Design review of the part built by this model. Coordinates are the model's own, in mm. Face numbers are marked on the shaded views. A direction names the side the tool comes from. Coordinates: 2 decimals unless noted, no trailing zeros. Write each loop counter-clockwise with the first axis right and the second up, starting at its lowest first coordinate (ties: lowest second). Pieces come first, ordered by that corner, then holes. Notation, with made-up numbers: M 12,62 L 17,62 A28 ccw 17,91 Z; hole C 82,-37.5 d6. An arc over 180 degrees is marked long. Return JSON: item names as keys, results as strings. Group by question number.
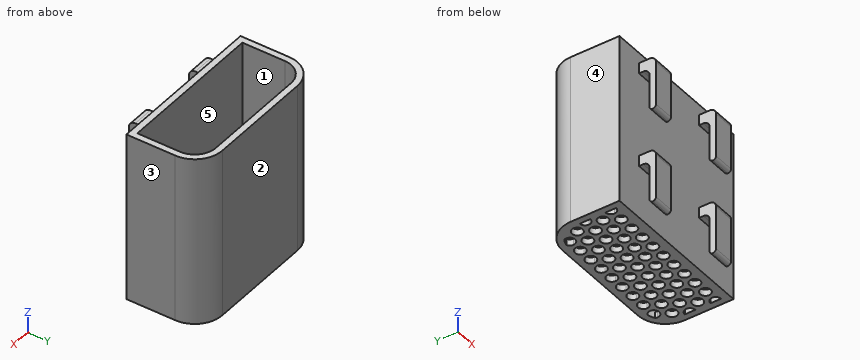
```python
from build123d import *

# Parameters (mm, degrees)
F1_DEPTH = 80
F2_DEPTH = 3
F3_R     = 2.5
F4_DEPTH = 3
F5_W     = 10
F5_H     = 5
F6_DEPTH = 5
F7_W     = 10
F7_H     = 25
F8_DEPTH = 3
F9_R     = 3
F10_R    = 1.49999


# Not quite as in the source:
# - a fillet or chamfer is up to 0.001 mm smaller than in the source, because OpenCascade refuses the exact size


with BuildPart() as f1:
    # F0 (on Top) → F1 (new body)
    with BuildSketch(Plane.XY):
        with BuildLine():
            Line((-38, 5), (-38, -18))
            Line((-38, -18), (38, -18))
            Line((38, -18), (38, 5))
            ThreePointArc((38, 5), (34.1923881554, 14.1923881554), (25, 18))
            Line((25, 18), (-25, 18))
            ThreePointArc((-25, 18), (-34.1923881554, 14.1923881554), (-38, 5))
        make_face()
        with BuildLine():
            Line((35, -15), (-35, -15))
            Line((-35, -15), (-35, 5))
            ThreePointArc((-35, 5), (-32.0710678119, 12.0710678119), (-25, 15))
            Line((-25, 15), (25, 15))
            ThreePointArc((25, 15), (32.0710678119, 12.0710678119), (35, 5))
            Line((35, 5), (35, -15))
        make_face(mode=Mode.SUBTRACT)
    extrude(amount=F1_DEPTH)

    # F0 (on Top) → F2 (join)
    with BuildSketch(Plane.XY):
        with BuildLine():
            Line((-35, 5), (-35, -15))
            Line((-35, -15), (35, -15))
            Line((35, -15), (35, 5))
            ThreePointArc((35, 5), (32.0710678119, 12.0710678119), (25, 15))
            Line((25, 15), (-25, 15))
            ThreePointArc((-25, 15), (-32.0710678119, 12.0710678119), (-35, 5))
        make_face()
    extrude(amount=F2_DEPTH)

    # F3 (on face) → F4 (cut)
    with BuildSketch(Plane.XY.offset(3)):
        with BuildLine():
            ThreePointArc((-30.2998951749, 13.4800419301), (-28.5001310143, 10.050537004), (-25.5, 12.5))
            ThreePointArc((-25.5, 12.5), (-25.9114746987, 13.8740677079), (-27.0104496527, 14.7958201389))
            ThreePointArc((-27.0104496527, 14.7958201389), (-28.7139067635, 14.2847669089), (-30.2998951749, 13.4800419301))
        make_face()
        with BuildLine():
            ThreePointArc((23.5, 12.5), (22.767766953, 14.267766953), (21, 15))
            ThreePointArc((21, 15), (19.232233047, 10.732233047), (23.5, 12.5))
        make_face()
        with BuildLine():
            ThreePointArc((16.5, 12.5), (15.767766953, 14.267766953), (14, 15))
            ThreePointArc((14, 15), (12.232233047, 10.732233047), (16.5, 12.5))
        make_face()
        with BuildLine():
            ThreePointArc((9.5, 12.5), (8.7677669588, 14.2677669471), (7.0000000165, 15))
            ThreePointArc((7.0000000165, 15), (5.2322330412, 10.7322330529), (9.5, 12.5))
        make_face()
        with BuildLine():
            ThreePointArc((2.5, 12.5), (1.7677669531, 14.2677669529), (3e-10, 15))
            ThreePointArc((3e-10, 15), (-1.7677669531, 10.7322330471), (2.5, 12.5))
        make_face()
        with BuildLine():
            ThreePointArc((-4.5, 12.5), (-5.2322330412, 14.2677669471), (-6.9999999835, 15))
            ThreePointArc((-6.9999999835, 15), (-8.7677669588, 10.7322330529), (-4.5, 12.5))
        make_face()
        with BuildLine():
            ThreePointArc((-11.5, 12.5), (-12.2322330423, 14.2677669482), (-13.9999999867, 15))
            ThreePointArc((-13.9999999867, 15), (-15.7677669577, 10.7322330518), (-11.5, 12.5))
        make_face()
        with BuildLine():
            ThreePointArc((-18.5, 12.5), (-19.232233047, 14.267766953), (-21, 15))
            ThreePointArc((-21, 15), (-22.767766953, 10.732233047), (-18.5, 12.5))
        make_face()
        with BuildLine():
            ThreePointArc((-32.5, 0.3621778265), (-33.232233047, 2.1299447795), (-35, 2.8621778265))
            Line((-35, 2.8621778265), (-35, -2.1378221735))
            ThreePointArc((-35, -2.1378221735), (-33.232233047, -1.4055891265), (-32.5, 0.3621778265))
        make_face()
        with BuildLine():
            ThreePointArc((-32.5, -11.775644347), (-33.232233047, -10.0078773941), (-35, -9.275644347))
            Line((-35, -9.275644347), (-35, -14.275644347))
            ThreePointArc((-35, -14.275644347), (-33.232233047, -13.5434113), (-32.5, -11.775644347))
        make_face()
        with BuildLine():
            ThreePointArc((35, -9.275644347), (32.5, -11.775644347), (35, -14.275644347))
            Line((35, -14.275644347), (35, -9.275644347))
        make_face()
        with BuildLine():
            ThreePointArc((30.2998951749, 13.4800419301), (28.7139067635, 14.2847669089), (27.0104496527, 14.7958201389))
            ThreePointArc((27.0104496527, 14.7958201389), (26.6259322921, 10.4114746987), (30.5, 12.5))
            ThreePointArc((30.5, 12.5), (30.449462996, 13.0001310143), (30.2998951749, 13.4800419301))
        make_face()
        with BuildLine():
            ThreePointArc((35, 2.8621778265), (32.5, 0.3621778265), (35, -2.1378221735))
            Line((35, -2.1378221735), (35, 2.8621778265))
        make_face()
        with Locations((10.5, 6.4378221735)):
            Circle(F3_R)
        with Locations((-24.5, 6.4378221735)):
            Circle(F3_R)
        with Locations((-3.5, 6.4378221735)):
            Circle(F3_R)
        with Locations((24.5, 6.4378221735)):
            Circle(F3_R)
        with Locations((-17.5, 6.4378221735)):
            Circle(F3_R)
        with Locations((17.5, 6.4378221735)):
            Circle(F3_R)
        with Locations((3.5, 6.4378221735)):
            Circle(F3_R)
        with Locations((-31.5, 6.4378221735)):
            Circle(F3_R)
        with Locations((31.5, 6.4378221735)):
            Circle(F3_R)
        with Locations((-10.5, 6.4378221735)):
            Circle(F3_R)
        with Locations((31.5, -5.7)):
            Circle(F3_R)
        with Locations((28, 0.3621778265)):
            Circle(F3_R)
        with Locations((-14, 0.3621778265)):
            Circle(F3_R)
        with Locations((-31.5, -5.7)):
            Circle(F3_R)
        with Locations((-7, 0.3621778265)):
            Circle(F3_R)
        with Locations((0, 0.3621778265)):
            Circle(F3_R)
        with Locations((10.5, -5.7)):
            Circle(F3_R)
        with Locations((-21, 0.3621778265)):
            Circle(F3_R)
        with Locations((-28, 0.3621778265)):
            Circle(F3_R)
        with Locations((-10.5, -5.7)):
            Circle(F3_R)
        with Locations((17.5, -5.7)):
            Circle(F3_R)
        with Locations((-24.5, -5.7)):
            Circle(F3_R)
        with Locations((7, 0.3621778265)):
            Circle(F3_R)
        with Locations((-3.5, -5.7)):
            Circle(F3_R)
        with Locations((24.5, -5.7)):
            Circle(F3_R)
        with Locations((14, 0.3621778265)):
            Circle(F3_R)
        with Locations((21, 0.3621778265)):
            Circle(F3_R)
        with Locations((3.5, -5.7)):
            Circle(F3_R)
        with Locations((-17.5, -5.7)):
            Circle(F3_R)
        with Locations((28, -11.775644347)):
            Circle(F3_R)
        with Locations((-14, -11.775644347)):
            Circle(F3_R)
        with Locations((-7, -11.775644347)):
            Circle(F3_R)
        with Locations((0, -11.775644347)):
            Circle(F3_R)
        with Locations((-21, -11.775644347)):
            Circle(F3_R)
        with Locations((-28, -11.775644347)):
            Circle(F3_R)
        with Locations((7, -11.775644347)):
            Circle(F3_R)
        with Locations((14, -11.775644347)):
            Circle(F3_R)
        with Locations((21, -11.775644347)):
            Circle(F3_R)
    extrude(amount=-F4_DEPTH, mode=Mode.SUBTRACT)

    # F5 (on face) → F6 (join)
    with BuildSketch(Plane.XZ.offset(18)):
        with Locations((-20, 72.5)):
            Rectangle(F5_W, F5_H)
        with Locations((20, 72.5)):
            Rectangle(F5_W, F5_H)
        with Locations((20, 27.5)):
            Rectangle(F5_W, F5_H)
        with Locations((-20, 27.5)):
            Rectangle(F5_W, F5_H)
    extrude(amount=F6_DEPTH)

    # F7 (on face) → F8 (join)
    with BuildSketch(Plane.XZ.offset(23)):
        with Locations((-20, 62.5)):
            Rectangle(F7_W, F7_H)
        with Locations((20, 62.5)):
            Rectangle(F7_W, F7_H)
        with Locations((20, 17.5)):
            Rectangle(F7_W, F7_H)
        with Locations((-20, 17.5)):
            Rectangle(F7_W, F7_H)
    extrude(amount=F8_DEPTH)

    # F9
    f9_edges = [f1.edges().sort_by_distance(p)[0] for p in [
        (-20, -26, 30),
        (20, -26, 30),
        (-20, -26, 75),
        (20, -26, 75),
        (20, -23, 25),
        (20, -23, 70),
        (-20, -23, 70),
        (-20, -23, 25),
    ]]
    fillet(f9_edges, radius=F9_R)

    # F10 (radius 1.5 in the source; OpenCascade refuses exactly that, so slightly less here)
    f10_edges = [f1.edges().sort_by_distance(p)[0] for p in [
        (20, -26, 50),
        (20, -23, 50),
        (20, -23, 5),
        (-20, -26, 50),
        (-20, -23, 50),
        (-20, -23, 5),
        (-20, -26, 5),
        (20, -26, 5),
    ]]
    fillet(f10_edges, radius=F10_R)


solid = f1.part
```
Item 1: For line 1 (Y direction, x = 14, z = 0.8); line 2 (Y direction, x = -10.5, z = 1.25); line 3 (Y direction, x = -22, z = 67), list the stretches that pass through material, from the lowest coordinate up.
Item 2: Add section A-A (z = 66). Write out the cut boundary in (x, y).
Item 3: Add section D-D (x = 28). Write out the cut boundary in (y, z).
Item 4: For pin 1 (2 mm diameter, centred on y = -20, z = 57, fed in from -X); pin 2 (10 mm diameter, centred on x = -6.5, y = 1, fed in from +Z); pin 3 (4 mm diameter, centred on y = -23.5, z = 59, fed in from +X); pin 4 (5 mm diameter, centred on x = -23.5, z = 48, fed in from -Y), all flat-tipped, find the tip position at first contact; note any pin that passes through.
Item 5: The part is to be moulded in two halves that separate along X. For the marked faces 1, 2 and 3, say which applies: pulls with the +X half, pulls with the -X half, needs draft (parallel to the pull), parting line crosses it, or undercut.
Item 6: Machinability: for the marked faces 4 and 5, which of the approach directions +Z, -Z, +X, -X, +Y, -Y give a long, thin tool a straight path to every point of the face, cutting with its end or side? Answer none if there is none.
Item 7: Add section B-B (x = -3.5). Write out the cut boundary in (y, z), plus the area to 3 significant figures.
Item 8: Add section C-C (z = 48.5). Write out the cut boundary in (x, y).
Geometry check:
{
 "1": {"line 1": "-18 to -14.28, -9.28 to -2.14, 2.86 to 10, 15 to 18", "line 2": "-18 to -8.2, -3.2 to 3.94, 8.94 to 18", "line 3": "-26 to -23, -18 to -15, 15 to 18"},
 "2": {"outline": "M -38,-18 L 38,-18 L 38,5 A13 ccw 25,18 L -25,18 A13 ccw -38,5 Z; M -25,-26 L -15,-26 L -15,-23 L -25,-23 Z; M 15,-26 L 25,-26 L 25,-23 L 15,-23 Z; hole M -35,-15 L 35,-15 L 35,5 A10 ccw 25,15 L -25,15 A10 ccw -35,5 Z"},
 "3": {"outline": "M -18,0 L -14.28,0 L -14.28,3 L -15,3 L -15,80 L -18,80 Z; M -9.28,0 L -2.14,0 L -2.14,3 L -9.28,3 Z; M 2.86,0 L 10,0 L 10,3 L 2.86,3 Z; M 14.54,0 L 17.65,0 L 17.65,80 L 14.54,80 Z"},
 "4": {"pin 1": "through", "pin 2": "z = 3", "pin 3": "x = 25", "pin 4": "y = -25.62"},
 "5": {"face 1": "undercut", "face 2": "needs draft", "face 3": "pulls with the +X half"},
 "6": {"face 4": "+Z, -Z, -X, +Y, -Y", "face 5": "+Z"},
 "7": {"outline": "M -18,0 L -8.2,0 L -8.2,3 L -15,3 L -15,80 L -18,80 Z; M -3.2,0 L 3.94,0 L 3.94,3 L -3.2,3 Z; M 8.94,0 L 18,0 L 18,80 L 15,80 L 15,3 L 8.94,3 Z", "area": "540 mm^2"},
 "8": {"outline": "M -38,-18 L 38,-18 L 38,5 A13 ccw 25,18 L -25,18 A13 ccw -38,5 Z; hole M -35,-15 L 35,-15 L 35,5 A10 ccw 25,15 L -25,15 A10 ccw -35,5 Z"}
}
